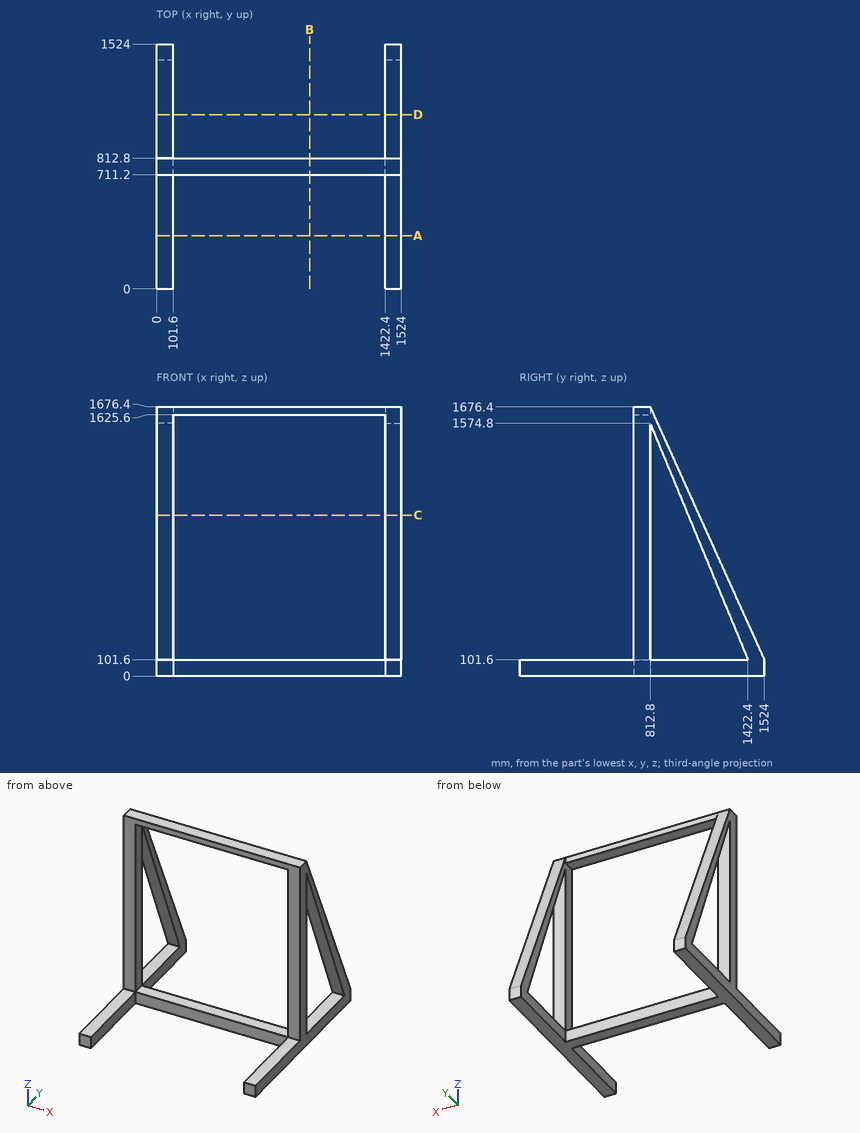
Check sheet for the drawn part. Datum: minimum x, y, z corner. Units: mm. Round coordinates to 2 decimals unless told otherwise and drop trailing zeros. Write each loop counter-clockwise with the first axis right and the second up, starting at its lowest first coordinate (ties: lowest second). Pieces come first, ordered by that corner, then holes. Notation, with made-up numbers: (-15.5, 58) -> (2.5, 58) arc R16 cw to (2.5, 65) -> close; hole circle Ø3 at (-6, 45). An arc over 180 degrees is marked (long way). Put each result on its own line as item: value.
(1) Sectioned sample at D-D (y = 1083.5). Enter the section's corners in (x, z).
Values found:
outline: (0, 0) -> (101.6, 0) -> (101.6, 101.6) -> (0, 101.6) -> close; (0, 920.61) -> (101.6, 920.61) -> (101.6, 1076.99) -> (0, 1076.99) -> close; (1422.4, 0) -> (1524, 0) -> (1524, 101.6) -> (1422.4, 101.6) -> close; (1422.4, 920.61) -> (1524, 920.61) -> (1524, 1076.99) -> (1422.4, 1076.99) -> close
(2) Sectioned sample at A-A (y = 330.5). Enter the section's corners in (x, z), plus the area to 3 significant figures.
Values found:
outline: (0, 0) -> (101.6, 0) -> (101.6, 101.6) -> (0, 101.6) -> close; (1422.4, 0) -> (1524, 0) -> (1524, 101.6) -> (1422.4, 101.6) -> close
area: 20,600 mm^2
(3) Material ranges on line 1 (X direction, y = 749.5, z = 125); line 2 (Y direction, x = 1458, z = 192.5); line 3 (Z direction, x = 351.5, y = 736.5), recorded low to high.
Values found:
line 1: x = 0 to 101.6, 1422.4 to 1524
line 2: y = 711.2 to 812.8, 1384.79 to 1482.95
line 3: z = 0 to 101.6, 1625.6 to 1676.4
(4) Sectioned sample at C-C (z = 1001.5). Enter the section's corners in (x, y), plus the area to 3 significant figures.
Values found:
outline: (0, 711.2) -> (101.6, 711.2) -> (101.6, 812.8) -> (0, 812.8) -> close; (0, 1050.03) -> (101.6, 1050.03) -> (101.6, 1117.59) -> (0, 1117.59) -> close; (1422.4, 711.2) -> (1524, 711.2) -> (1524, 812.8) -> (1422.4, 812.8) -> close; (1422.4, 1050.03) -> (1524, 1050.03) -> (1524, 1117.59) -> (1422.4, 1117.59) -> close
area: 34,400 mm^2
(5) Sectioned sample at B-B (x = 951.5). Enter the section's corners in (y, z).
Values found:
outline: (711.2, 0) -> (812.8, 0) -> (812.8, 101.6) -> (711.2, 101.6) -> close; (711.2, 1625.6) -> (812.8, 1625.6) -> (812.8, 1676.4) -> (711.2, 1676.4) -> close
